from build123d import *

# Parameters (mm, degrees)
SKETCH_1_W          = 75
SKETCH_1_H          = 110
EXTRUDE_1_DEPTH     = 5
SKETCH_2_W          = 65
SKETCH_2_H          = 5
SKETCH_2_W_2        = 56
EXTRUDE_2_DEPTH     = 23
SKETCH_3_R          = 1.5
SKETCH_3_W          = 23
SKETCH_3_H          = 13
CUT_EXTRUDE_1_DEPTH = 10
CUT_EXTRUDE_2_REACH = 120.34
SKETCH_5_W          = 16
SKETCH_5_H          = 20
CUT_EXTRUDE_3_REACH = 120.34
SKETCH_6_R          = 1.5
CUT_EXTRUDE_4_REACH = 124.798
SKETCH_7_R          = 1.5
SKETCH_8_W          = 5
SKETCH_8_H          = 80
EXTRUDE_3_DEPTH     = 6


with BuildPart() as part:
    # 草圖1 → 填料-伸長1 (new body)
    with BuildSketch(Plane.XY):
        with Locations((9.355675066, -19.631766382)):
            Rectangle(SKETCH_1_W, SKETCH_1_H)
    extrude(amount=EXTRUDE_1_DEPTH)

    # 草圖2 → 填料-伸長2 (add)
    with BuildSketch(Plane.XY.offset(5)):
        with Locations((9.355675066, -72.131766382)):
            Rectangle(SKETCH_2_W, SKETCH_2_H)
        with Locations((13.855675066, 32.868233618)):
            Rectangle(SKETCH_2_W_2, SKETCH_2_H)
    extrude(amount=EXTRUDE_2_DEPTH)

    # 草圖3 → 除料-伸長1 (cut)
    with BuildSketch(Plane(origin=(0, 35.368233618, 0), x_dir=(1, 0, 0), z_dir=(0, 1, 0))):
        with Locations(Location((2.855675066, -16, 0), (0, 0, 270))):
            Circle(SKETCH_3_R)
        with Locations(Location((-8.144324934, -16, 0), (0, 0, 270))):
            Circle(SKETCH_3_R)
        with Locations((20.355675066, -21.5)):
            Rectangle(SKETCH_3_W, SKETCH_3_H)
    extrude(amount=-CUT_EXTRUDE_1_DEPTH, mode=Mode.SUBTRACT)

    # 草圖5 → 除料-伸長2 (cut, up to next)
    with BuildSketch(Plane(origin=(0, -69.631766382, 0), x_dir=(1, 0, 0), z_dir=(0, 1, 0)), mode=Mode.PRIVATE) as cut_extrude_2_sk1:
        with Locations((15.855675066, -18)):
            Rectangle(SKETCH_5_W, SKETCH_5_H)
    cut_extrude_2_tool1 = extrude(cut_extrude_2_sk1.sketch, amount=-CUT_EXTRUDE_2_REACH, mode=Mode.PRIVATE) & part.part
    add(cut_extrude_2_tool1.solids().sort_by_distance((15.855675, -69.631766, 18))[0], mode=Mode.SUBTRACT)

    # 草圖6 → 除料-伸長3 (cut, up to next)
    with BuildSketch(Plane(origin=(0, -69.631766382, 0), x_dir=(1, 0, 0), z_dir=(0, 1, 0)), mode=Mode.PRIVATE) as cut_extrude_3_sk1:
        with Locations(Location((31.855675066, -16, 0), (0, 0, 270))):
            Circle(SKETCH_6_R)
    cut_extrude_3_tool1 = extrude(cut_extrude_3_sk1.sketch, amount=-CUT_EXTRUDE_3_REACH, mode=Mode.PRIVATE) & part.part
    add(cut_extrude_3_tool1.solids().sort_by_distance((31.855675, -69.631766, 16))[0], mode=Mode.SUBTRACT)

    # 草圖7 → 除料-伸長4 (cut, up to next)
    with BuildSketch(Plane.XZ.offset(74.631766382), mode=Mode.PRIVATE) as cut_extrude_4_sk1:
        with Locations(Location((-7.144324934, 16, 0), (0, 0, 270))):
            Circle(SKETCH_7_R)
    cut_extrude_4_tool1 = extrude(cut_extrude_4_sk1.sketch, amount=-CUT_EXTRUDE_4_REACH, mode=Mode.PRIVATE) & part.part
    add(cut_extrude_4_tool1.solids().sort_by_distance((-7.144325, -74.631766, 16))[0], mode=Mode.SUBTRACT)

    # 草圖8 → 填料-伸長3 (add)
    with BuildSketch(Plane.XY.offset(5)):
        with Locations((-20.644324934, -29.631766382)):
            Rectangle(SKETCH_8_W, SKETCH_8_H)
    extrude(amount=EXTRUDE_3_DEPTH)


solid = part.part
Part model, mm, in its own coordinate system. A direction names the side the tool comes from. Coordinates: 2 decimals unless noted, no trailing zeros. Loops run counter-clockwise (first coordinate to the right, second up) from the corner with the lowest first, then second, coordinate; pieces in that order, holes last. Notation, with made-up numbers: M 51,23 L 101,23 A29 ccw 101,46 Z; hole C 4.5,-33.5 d11. An arc over 180 degrees is marked long. Use a Markdown table: item, result. Add a question column.
Q1. Cut at A-A (y = -33). Write the cut outline in (x, z).
Q2. Which spindle directions (+Z, -Z, +X, -X, +Y, -Y) get a long thin tool onto all of the face, cutting with end or side? Do faces 1 (the cylindrical face through (2.9, 32.9, 14.5)), 2 (the flat face through (8.856, 33, 22)), 3 (the flat face through (-18.144, -30, 8)), 4 (the flat face through (41.856, -72, 16)), 5 (the flat face through (-21, 10.368, 8)). Say none if no direction does.
Q3. Pin check, flat tips, straight feed: P1, Ø4, axis at y = 34, z = 18, coming from the -X side; P2, Ø1.8, axis at x = -8.14, z = 16, coming from the +Y side; P3, Ø2.5, axis at x = 25.5, y = 33.5, coming from the +Z side. Stop position of each tip, or through.
Q4. Mould opens along X. For faces 6 (the flat face through (31.856, 33, 22)), 7 (the flat face through (41.856, 33, 16)), 8 (the flat face through (8.8, -74.632, 7.6)), 9 (the flat face through (-23.144, -39, 10)) say: +X half, -X half, draft (parallel to the pull), parting line (faces both ways), or undercut.
Q5. Cut at B-B (x = 26.5). Write the cut outline in (y, z), and give its area (3 significant figures).
Q6. Cut at C-C (z = 16.25). Give the number of separate pieces and of enclosed holes in the cut face, and give its area (3 significant figures).
Q7. Probe L1, parallel to Y at x = 37, z = 5.75; L2, parallel to X at y = -70.95, z = 16; L3, parallel to Y at x = 16, z = 14. List the from-to ranges inside material, lowest first.
Worked out:
| question | item | result |
|---|---|---|
| 1 | outline | M -28.14,0 L 46.86,0 L 46.86,5 L -18.14,5 L -18.14,11 L -23.14,11 L -23.14,5 L -28.14,5 Z |
| 2 | face 1 | +Y |
| 2 | face 2 | +Z, +Y, -Y |
| 2 | face 3 | +Z, +X, +Y |
| 2 | face 4 | +Z, +X, +Y, -Y |
| 2 | face 5 | +Z, +X, -X, +Y |
| 3 | P1 | stops at x = -14.14 |
| 3 | P2 | stops at y = -69.63 |
| 3 | P3 | stops at z = 15 |
| 4 | face 6 | undercut |
| 4 | face 7 | +X half |
| 4 | face 8 | draft |
| 4 | face 9 | -X half |
| 5 | outline | M -74.63,0 L 35.37,0 L 35.37,15 L 30.37,15 L 30.37,5 L -69.63,5 L -69.63,28 L -74.63,28 Z |
| 5 | area | 715 mm2 |
| 6 | separate pieces | 8 |
| 6 | enclosed holes | 0 |
| 6 | area | 351 mm2 |
| 7 | L1 | y = -74.63 to -69.63, 30.37 to 35.37 |
| 7 | L2 | x = -23.14 to -8.64, -5.64 to 7.86, 23.86 to 30.36, 33.36 to 41.86 |
| 7 | L3 | y = 30.37 to 35.37 |
